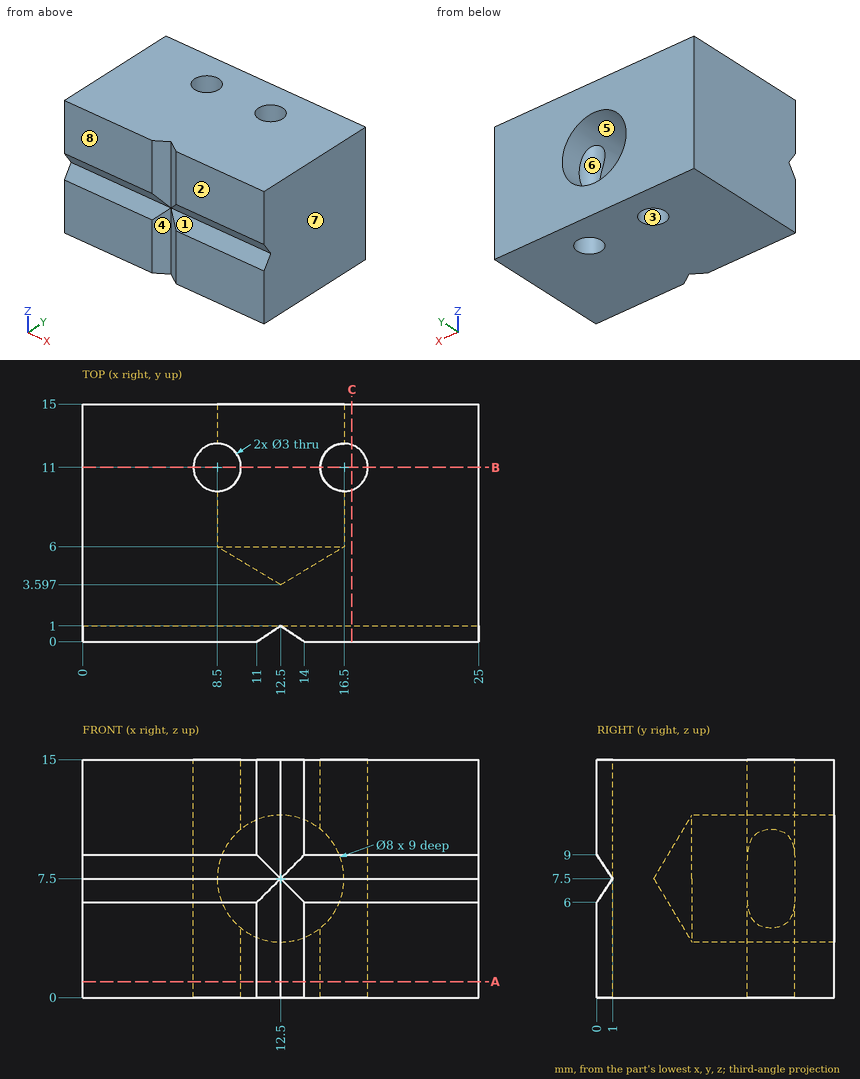
Could you check a few things on this drawing? It's one solid part, dimensions in mm from its lowest x, y, z. A direction names the side the tool comes from. Coordinates: 2 decimals unless noted, no trailing zeros. Write each loop counter-clockwise with the first axis right and the second up, starting at its lowest first coordinate (ties: lowest second). Pieces come first, ordered by that corner, then holes. Notation, with made-up numbers: (-28.75, -17.75) - (24.25, -17.75) arc R23 cw to (24.25, 17.25) - close; hole circle Ø3 at (1, 87). An arc over 180 degrees is marked (long way). Return JSON: item names as keys, results as strings. Group by question number.
Item 1: We'd pull the mould along X, two halves only. Please class the marked faces 6, 7 and 8: pulls with the +X half, pulls with the -X half, needs draft (parallel to the pull), parting line crosses it, or undercut.
Item 2: If we section it at C-C (x = 17): Write out the boundary of the cut face in (y, z) (1 decimal), then the cut area to 3 significant figures.
Item 3: If we section it at A-A (z = 1): Write out the boundary of the cut face in (x, y), then the cut area to 3 significant figures.
Item 4: If we section it at B-B (y = 11): Write out the boundary of the cut face in (x, z).
Item 5: Please list where these lines run through material, in increasing order: probe 1 along Y at (x, z) = (8.5, 9.25); probe 2 along Z at (x, y) = (12.5, 11.5); probe 3 along Y at (x, z) = (16.5, 7) (1 decimal).
Item 6: I'm going to push flat-ended pins straight in: pin 1 Ø2.5 at (x, y) = (16.5, 11) entering from -Z; pin 2 Ø2 at (x, z) = (15, 7.5) entering from +Y. Where does each tip first touch, or does it pass through?
Item 7: Which directions (+Z, -Z, +X, -X, +Y, -Y) give clear straight access to the entire face, cutting with the end or side of a thin tool? Please do the marked faces 1, 2, 3, 4 and 5.
Return value:
{
 "1": {"face 6": "undercut", "face 7": "pulls with the +X half", "face 8": "needs draft"},
 "2": {"outline": "(0, 0) - (9.6, 0) - (9.6, 15) - (0, 15) - (0, 9) - (1, 7.5) - (0, 6) - close; (12.4, 0) - (15, 0) - (15, 15) - (12.4, 15) - close", "area": "181 mm^2"},
 "3": {"outline": "(0, 0) - (11, 0) - (12.5, 1) - (14, 0) - (25, 0) - (25, 15) - (0, 15) - close; hole circle Ø3 at (8.5, 11); hole circle Ø3 at (16.5, 11)", "area": "359 mm^2"},
 "4": {"outline": "(0, 0) - (7, 0) - (7, 15) - (0, 15) - close; (10, 0) - (15, 0) - (15, 4.38) arc R4 cw to (10, 4.38) - close; (10, 10.62) arc R4 cw to (15, 10.62) - (15, 15) - (10, 15) - close; (18, 0) - (25, 0) - (25, 15) - (18, 15) - close"},
 "5": {"probe 1": "y = 0 to 9.5, 12.5 to 15", "probe 2": "z = 0 to 3.5, 11.5 to 15", "probe 3": "y = 0.7 to 9.5, 12.5 to 15"},
 "6": {"pin 1": "passes through", "pin 2": "stops at y = 5.7"},
 "7": {"face 1": "+X, -X, -Y", "face 2": "+Z, -Z, +X, -X, -Y", "face 3": "+Z, -Z", "face 4": "+Z, -Z, -Y", "face 5": "+Y"}
}
